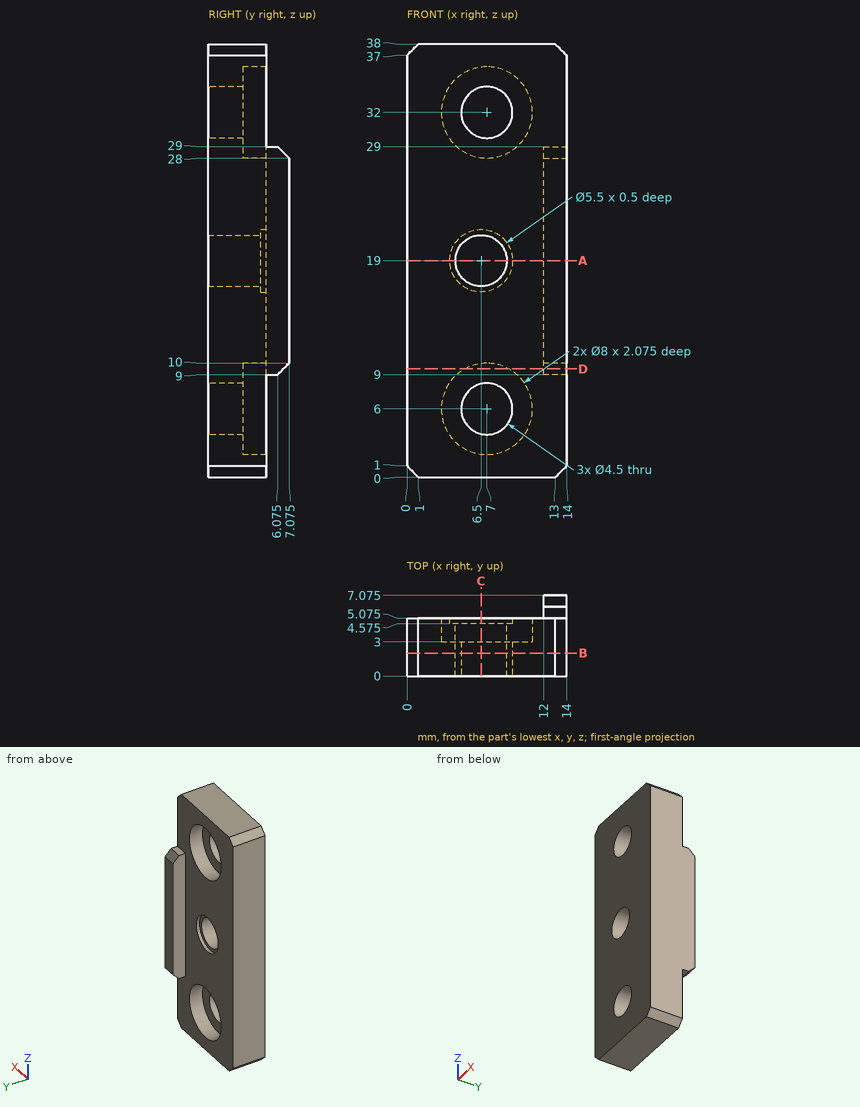
Study the drawing (mm; zero at the part's minimum x, y, z) and answer. Give positions to 0.01 mm unless a question says otherwise; leave off trailing zeros. Write each loop counter-clockwise with the first axis right and the second up, starting at its lowest first coordinate (ties: lowest second). Pieces come first, ordered by that corner, then holes. Notation, with made-up numbers: (54.5, 70) - (66.5, 70) arc R18 cw to (66.5, 75) - close; hole circle Ø7 at (-16, -12.75). An arc over 180 degrees is marked (long way). One line per question, with ' | ' between items. Start each with the question number.
1. Straight lines are drawn through the part: line 1 (Z direction, x = 5.25, y = 4); line 2 (X direction, y = 4.95, z = 19); line 3 (Z direction, x = 7, y = 1.95). For each, find the intervals that lie inside material, in ascending order.
2. Section A-A, the plane z = 19 is taken. Determine the outline of the cut face in (x, y) (3 decimals), then the cut area to 3 significant figures.
3. Section C-C, the plane x = 6.5 is taken. Determine the outline of the cut face in (y, z) (3 decimals), then the cut area to 3 significant figures.
4. Given P1, Ø1.6, axis at x = 6.5, z = 18, coming from the +Y side; P2, Ø1.5, axis at x = 3.5, z = 27, coming from the +Y side (3 decimals); P3, Ø6.5, axis at x = 7, z = 32, coming from the +Y side; P4, Ø0.5, axis at x = 12.5, y = 6, coming from the +Z side, each flat-ended and moving along its own axis, determine where each tip first touches the part or whether it passes through.
5. Section B-B, the plane y = 2 is taken. Determine the outline of the cut face in (x, z).
6. Section D-D, the plane z = 9.5 is taken. Determine the outline of the cut face in (x, y) (1 decimal), then the cut area to 3 significant figures.
Result:
1) line 1: z = 0 to 2.4, 9.6 to 17.13, 20.87 to 28.4, 35.6 to 38 | line 2: x = 0 to 3.75, 9.25 to 14 | line 3: z = 0 to 3.75, 8.25 to 16.81, 21.19 to 29.75, 34.25 to 38
2) outline: (0, 0) - (4.25, 0) - (4.25, 4.575) - (3.75, 4.575) - (3.75, 5.075) - (0, 5.075) - close; (8.75, 0) - (14, 0) - (14, 7.075) - (12, 7.075) - (12, 5.075) - (9.25, 5.075) - (9.25, 4.575) - (8.75, 4.575) - close | area: 51.7 mm2
3) outline: (0, 0) - (5.075, 0) - (5.075, 2.031) - (3, 2.031) - (3, 3.806) - (0, 3.806) - close; (0, 8.194) - (3, 8.194) - (3, 9.969) - (5.075, 9.969) - (5.075, 16.25) - (4.575, 16.25) - (4.575, 16.75) - (0, 16.75) - close; (0, 21.25) - (4.575, 21.25) - (4.575, 21.75) - (5.075, 21.75) - (5.075, 28.031) - (3, 28.031) - (3, 29.806) - (0, 29.806) - close; (0, 34.194) - (3, 34.194) - (3, 35.969) - (5.075, 35.969) - (5.075, 38) - (0, 38) - close | area: 110 mm2
4) P1: passes through | P2: stops at y = 5.075 | P3: stops at y = 3 | P4: stops at z = 29
5) outline: (0, 1) - (1, 0) - (13, 0) - (14, 1) - (14, 37) - (13, 38) - (1, 38) - (0, 37) - close; hole circle Ø4.5 at (6.5, 19); hole circle Ø4.5 at (7, 6); hole circle Ø4.5 at (7, 32)
6) outline: (0, 0) - (14, 0) - (14, 6.6) - (12, 6.6) - (12, 5.1) - (8.9, 5.1) - (8.9, 3) - (5.1, 3) - (5.1, 5.1) - (0, 5.1) - close | area: 66.0 mm2
